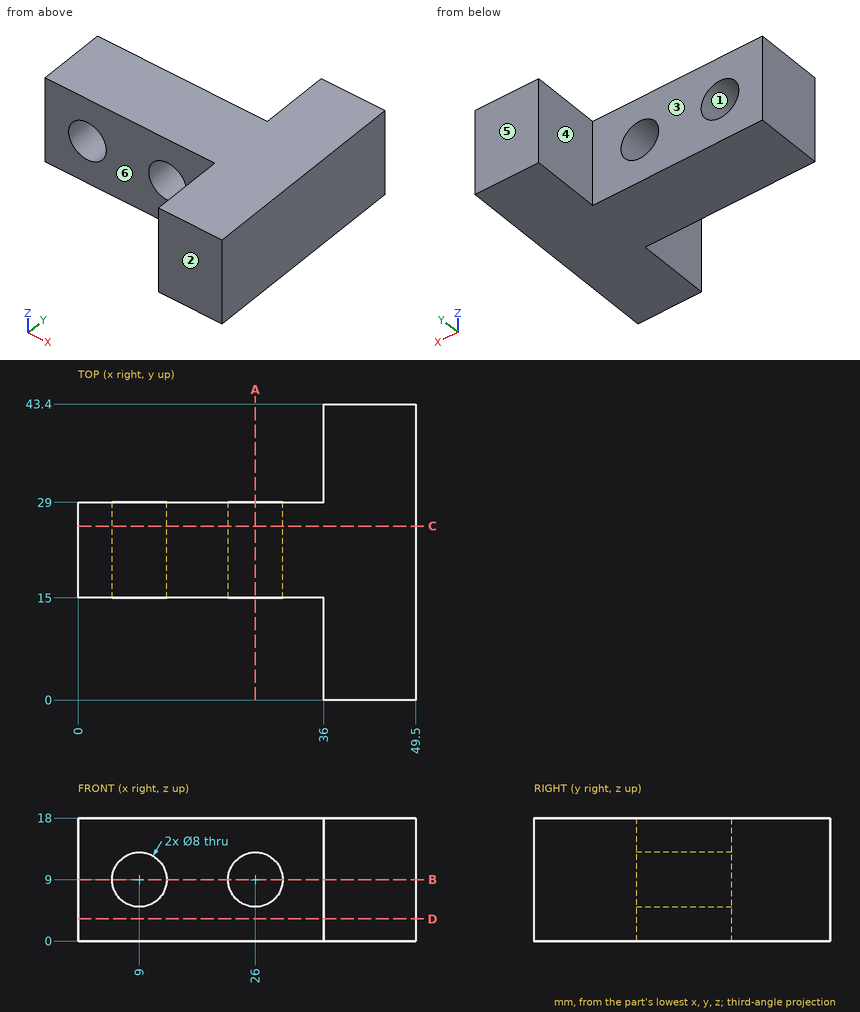
Can you work these out from the drawing? Everything is in mm from the part's minimum corner. A direction names the side the tool comes from. Give positions to 0.01 mm unless a question says otherwise; leave off trailing zeros. Order: outer loops, then holes, each group sorted by start corner. A loop starts at its lowest first (then second) coordinate and runs counter-clockwise, first axis right, second up. Notation, with made-up numbers: M 61.25,69 L 95.25,69 A22 cw 95.25,76 Z; hole C 57.25,-28.5 d5. An arc over 180 degrees is marked long. One line per item, written item: value.
Item 1: If we section it at C-C on y = 25.5: Write out the boundary of the cut face in (x, z), and give its area (3 significant figures).
Verdict:
outline: M 0,0 L 49.5,0 L 49.5,18 L 0,18 Z; hole C 9,9 d8; hole C 26,9 d8
area: 790 mm2
Item 2: Please list where these lines run through material, in increasing order: line 1 (X direction, y = 23.75, z = 9); line 2 (X direction, y = 32.5, z = 17); line 3 (Y direction, x = 2.5, z = 15.5).
Verdict:
line 1: 0 to 5, 13 to 22, 30 to 49.5
line 2: 36 to 49.5
line 3: 15 to 29
Item 3: For pin 1 (8 mm diameter, centred on x = 24.5, z = 15.5, fed in from -Y); pin 2 (10 mm diameter, centred on x = 12.5, z = 9.5, fed in from +Y); pin 3 (1 mm diameter, centred on y = 39, z = 4.5, fed in from -X), each with a flat end and sliding along its axis, tell me the tip position at first contact or that it passes through.
Verdict:
pin 1: y = 15
pin 2: y = 29
pin 3: x = 36
Item 4: If we section it at B-B on z = 9: Write out the boundary of the cut face in (x, y), and give its area (3 significant figures).
Verdict:
outline: M 0,15 L 5,15 L 5,29 L 0,29 Z; M 13,15 L 22,15 L 22,29 L 13,29 Z; M 30,15 L 36,15 L 36,0 L 49.5,0 L 49.5,43.4 L 36,43.4 L 36,29 L 30,29 Z
area: 866 mm2
Item 5: If we section it at D-D on z = 3.25: Write out the boundary of the cut face in (x, y), and give its area (3 significant figures).
Verdict:
outline: M 0,15 L 36,15 L 36,0 L 49.5,0 L 49.5,43.4 L 36,43.4 L 36,29 L 0,29 Z
area: 1,090 mm2
Item 6: For the marked faces 4, 5 and 6, which set-ups out of +Z, -Z, +X, -X, +Y, -Y let a thin tool reach every point of the face, with its end or its side?
Verdict:
face 4: +Z, -Z, -X, +Y
face 5: +Z, -Z, +X, -X, +Y
face 6: +Z, -Z, -X, -Y
Item 7: If we section it at A-A on x = 26: Write out the boundary of the cut face in (y, z).
Verdict:
outline: M 15,0 L 29,0 L 29,5 L 15,5 Z; M 15,13 L 29,13 L 29,18 L 15,18 Z
Item 8: If we mould it in two halves opening along Y, with no side actions, what happens to the marked faces 1, 2 and 3? For each: pulls with the +Y half, pulls with the -Y half, needs draft (parallel to the pull), parting line crosses it, or undercut.
Verdict:
face 1: needs draft
face 2: pulls with the -Y half
face 3: pulls with the +Y half
